Input: part model. Units: mm. Frame: model coordinates. A direction names the side the tool comes from. Coordinates: 2 decimals unless noted, no trailing zeros. Write each loop counter-clockwise with the first axis right and the second up, starting at its lowest first coordinate (ties: lowest second). Pieces come first, ordered by that corner, then holes. Notation, with made-up numbers: (55, 2.5) - (108, 2.5) arc R11 cw to (108, 20.5) - close; hole circle Ø10 at (-14.5, 60.25). An arc over 180 degrees is marked (long way). Use CSV: the item, a comma, the result in double quotes.
Autodesk Inventor part; units mm, degrees
ref_plane "YZ Plane" through (0, 0, 0) normal (1, 0, 0) x (0, 1, 0)
ref_plane "XZ Plane" through (0, 0, 0) normal (0, 1, 0) x (-1, 0, 0)
ref_plane "XY Plane" through (0, 0, 0) normal (0, 0, 1) x (1, 0, 0)
sketch "Sketch1" plane through (0, 0, 0) normal (0, 0, 1) x (1, 0, 0)
  line L0 (0, 0) -> (812.8, 0) construction
  line L1 (812.8, 0) -> (812.8, -406.4) construction
  line L2 (812.8, -406.4) -> (0, -406.4) construction
  line L3 (0, -406.4) -> (0, 0) construction
  line L4 (0, 0) -> (406.4, 0)
  line L5 (406.4, 0) -> (406.4, -25.4)
  line L6 (406.4, -25.4) -> (0, -25.4)
  line L7 (0, -25.4) -> (0, 0)
  line L8 (406.4, -25.4) -> (381, -25.4)
  line L9 (381, -25.4) -> (381, -406.4)
  line L10 (381, -406.4) -> (406.4, -406.4)
  line L11 (406.4, -406.4) -> (406.4, -25.4)
  line L12 (381, -406.4) -> (0, -406.4)
  line L13 (0, -406.4) -> (0, -381)
  line L14 (0, -381) -> (381, -381)
  line L15 (381, -381) -> (381, -406.4)
  line L16 (0, -381) -> (25.4, -381)
  line L17 (25.4, -381) -> (25.4, -25.4)
  line L18 (25.4, -25.4) -> (0, -25.4)
  line L19 (0, -25.4) -> (0, -381)
  dimension "d1" = 812.8
  dimension "d5" = 406.4
  dimension "d6" = 25.4
  dimension "d7" = 25.4
  dimension "d8" = 381
  dimension "d9" = 381
  dimension "d10" = 25.4
  dimension "d11" = 25.4
extrude "Extrusion1" add sketch "Sketch1" against normal blind 25.4 contours L6 L9 L14 L17
sketch "Sketch3" plane through (0, 0, 0) normal (0, 0, 1) x (1, 0, 0)
  line L0 (-406.4, 0) -> (406.4, 0) construction
  line L1 (406.4, 0) -> (406.4, -406.4) construction
  line L2 (406.4, -406.4) -> (-406.4, -406.4) construction
  line L3 (-406.4, -406.4) -> (-406.4, 0) construction
  line L4 (406.4, 0) -> (406.4, -406.4)
  line L5 (381, -381) -> (25.4, -381)
  line L6 (203.2, -381) -> (203.2, -355.6)
  line L7 (203.2, -355.6) -> (254, -355.6)
  line L8 (254, -355.6) -> (254, -50.8)
  line L9 (254, -50.8) -> (152.4, -50.8)
  line L10 (152.4, -50.8) -> (152.4, -355.6)
  line L11 (152.4, -355.6) -> (203.2, -355.6)
  point P0 (0, 0)
  dimension "d36" = 812.8
  dimension "d45" = 25.4
  dimension "d46" = 50.8
  dimension "d47" = 304.8
  dimension "d48" = 101.6
extrude "Extrusion3" cut sketch "Sketch3" against normal blind 25.4
properties part number "JukeBox Top Panel SQ"
(1) Ray query, probe 1 along X at (y, z) = (-137, -18); probe 2 along Y at (x, z) = (196.5, -13.75). Return the intervals inside material, ascending. Write a range as from..to.
Check values:
probe 1,"25.4..152.4, 254..381"
probe 2,"-381..-355.6, -50.8..-25.4"
(2) Draft query along X for faces 1 (the flat face through (152.4, -201, -13)), 2 (the flat face through (25.4, -206, -13)), 3 (the flat face through (280, -201, -25.4)). Return one class per face: pulls with the +X half, pulls with the -X half, needs draft (parallel to the pull), parting line crosses it, or undercut.
Check values:
face 1,"undercut"
face 2,"pulls with the -X half"
face 3,"needs draft"
(3) Cut plane A-A on y = -300.5. Return loops of the section in (x, z), and give its area (3 significant figures).
Check values:
outline,"(25.4, -25.4) - (152.4, -25.4) - (152.4, 0) - (25.4, 0) - close; (254, -25.4) - (381, -25.4) - (381, 0) - (254, 0) - close"
area,"6,450 mm^2"
(4) Reachability of faces 4 (the flat face through (254, -205, -13)), 5 (the flat face through (206, -25.4, -13)) from +Z, -Z, +X, -X, +Y, -Y: full face, straight path, thin tool, end or side. Return the list, or none.
Check values:
face 4,"+Z, -Z"
face 5,"+Z, -Z, +X, -X, +Y"
(5) Cut plane B-B on z = -4.5. Return loops of the section in (x, y), and give its area (3 significant figures).
Check values:
outline,"(25.4, -381) - (381, -381) - (381, -25.4) - (25.4, -25.4) - close; hole (152.4, -355.6) - (254, -355.6) - (254, -50.8) - (152.4, -50.8) - close"
area,"95,500 mm^2"
